```python
from build123d import *

# Parameters (mm, degrees)
SKETCH001_R   = 7
SKETCH001_R_2 = 30
PAD_DEPTH     = 18.5


with BuildPart() as part:
    # Sketch001 → Pad (new body)
    with BuildSketch(Plane.XY):
        with BuildLine():
            ThreePointArc((-51.0032, 68), (-63.021753, 63.021753), (-68, 51.0032))
            Line((-68, -51.0032), (-68, 51.0032))
            ThreePointArc((-68, -51.0032), (-63.021753, -63.021753), (-51.0032, -68))
            Line((51.0032, -68), (-51.0032, -68))
            ThreePointArc((51.0032, -68), (63.021753, -63.021753), (68, -51.0032))
            Line((68, 51.0032), (68, -51.0032))
            ThreePointArc((68, 51.0032), (63.021753, 63.021753), (51.0032, 68))
            Line((-51.0032, 68), (51.0032, 68))
        make_face()
        with Locations((51.0032, 51.0032)):
            Circle(SKETCH001_R, mode=Mode.SUBTRACT)
        with Locations((-51.0032, 51.0032)):
            Circle(SKETCH001_R, mode=Mode.SUBTRACT)
        with Locations((-51.0032, -51.0032)):
            Circle(SKETCH001_R, mode=Mode.SUBTRACT)
        with Locations((51.0032, -51.0032)):
            Circle(SKETCH001_R, mode=Mode.SUBTRACT)
        Circle(SKETCH001_R_2, mode=Mode.SUBTRACT)
    extrude(amount=PAD_DEPTH)


solid = part.part
```
Input: part model. Units: mm. Frame: model coordinates. Coordinates: 2 decimals unless noted, no trailing zeros. Loops run counter-clockwise (first coordinate to the right, second up) from the corner with the lowest first, then second, coordinate; pieces in that order, holes last. Notation, with made-up numbers: M 27,-30 L 54,-30 A18 ccw 54,-23 Z; hole C 68,49.25 d2. An arc over 180 degrees is marked long. Use a Markdown table: item, result. Add a question column.
1) Section A-A, the plane y = 0. Return the cut outline in (x, z), plus the area to 3 significant figures.
2) Section B-B, the plane z = 9.25. Return the cut outline in (x, y), plus the area to 3 significant figures.
3) Draft query along Y for faces 1 (the flat face through (-31, 1, 0)), 2 (the flat face through (1, -68, 9)), 3 (the cylindrical face through (-29.97, 1.32, 9.12)), 4 (the flat face through (-1, 68, 9)). Return one class per face: +Y half, -Y half, draft (parallel to the pull), parting line (faces both ways), or undercut.
4) Pin query (flat end, axial travel): P1, Ø11, axis at x = -51, y = -51, coming from the +Z side. Return the tip coordinate at first contact, or that it passes through.
5) Line query: L1, parallel to Y at x = 0, z = 4; L2, parallel to X at y = -49, z = 8; L3, parallel to Y at x = 55, z = 2. Output: solid intervals per line, ascending. Write a range as from..to.
Answer below:
| question | item | result |
|---|---|---|
| 1 | outline | M -68,0 L -30,0 L -30,18.5 L -68,18.5 Z; M 30,0 L 68,0 L 68,18.5 L 30,18.5 Z |
| 1 | area | 1,410 mm2 |
| 2 | outline | M -68,-51 A17 ccw -51,-68 L 51,-68 A17 ccw 68,-51 L 68,51 A17 ccw 51,68 L -51,68 A17 ccw -68,51 Z; hole C -51,-51 d14; hole C -51,51 d14; hole C 0,0 d60; hole C 51,-51 d14; hole C 51,51 d14 |
| 2 | area | 14,800 mm2 |
| 3 | face 1 | draft |
| 3 | face 2 | -Y half |
| 3 | face 3 | undercut |
| 3 | face 4 | +Y half |
| 4 | P1 | through |
| 5 | L1 | -68..-30, 30..68 |
| 5 | L2 | -68..-57.71, -44.3..44.3, 57.71..68 |
| 5 | L3 | -67.52..-56.75, -45.26..45.26, 56.75..67.52 |
